Verification items for the finished model (mm, model axes). Give positions to 0.01 mm unless a question says otherwise; leave off trailing zeros. Write each loop counter-clockwise with the first axis right and the second up, starting at its lowest first coordinate (ties: lowest second). Pieces come first, ordered by that corner, then holes.
from build123d import *

# Parameters (mm, degrees)
SKETCH1_W           = 52.3875
SKETCH1_H           = 52.3875
SKETCH1_R           = 9.525
BOSS_EXTRUDE1_DEPTH = 23.8125
FILLET1_R           = 2.54


with BuildPart() as part:
    # Sketch1 → Boss-Extrude1 (new body)
    with BuildSketch(Plane(origin=(0, 0, 0), x_dir=(1, 0, 0), z_dir=(0, 1, 0))):
        Rectangle(SKETCH1_W, SKETCH1_H)
        with Locations(Location((0, 0, 0), (0, 0, 270))):
            Circle(SKETCH1_R, mode=Mode.SUBTRACT)
    extrude(amount=BOSS_EXTRUDE1_DEPTH)

    # Fillet1
    fillet1_edges = [part.edges().sort_by_distance(p)[0] for p in [
        (26.19375, 23.8125, 0),
        (0, 23.8125, -9.525),
        (0, 23.8125, -26.19375),
        (-26.19375, 23.8125, 0),
        (0, 23.8125, 26.19375),
    ]]
    fillet(fillet1_edges, radius=FILLET1_R)


solid = part.part
Item 1: Sectioned sample at C-C on y = 3.5. Record the cut outline in (x, z) (3 decimals).
Answer key:
outline: (-26.194, -26.194) - (26.194, -26.194) - (26.194, 26.194) - (-26.194, 26.194) - close; hole circle Ø19.05 at (0, 0)
Item 2: Sectioned sample at D-D on y = 22. Record the cut outline in (x, z).
Answer key:
outline: (-26.09, -26.09) - (26.09, -26.09) - (26.09, 26.09) - (-26.09, 26.09) - close; hole circle Ø19.26 at (0, 0)
Item 3: Release check for a two-part mould opening along X. For faces 1 (the face through (11, 0, 0)), 2 (the face through (26.194, 10, 0)), 3 (the face through (-5.796, 10.487, -7.559)) record: released by +X, released by -X, zero draft, split by the parting line, or undercut.
Answer key:
face 1: zero draft
face 2: released by +X
face 3: undercut
Item 4: Scan lines: line 1 along X through (y, z) = (5.25, 0) (3 decimals); line 2 along X through (y, z) = (21.5, -16.5); line 3 along X through (y, z) = (23, 6.5). Record each from-to range of solid material in increasing order.
Answer key:
line 1: x = -26.194 to -9.525, 9.525 to 26.194
line 2: x = -26.18 to 26.18
line 3: x = -25.52 to -7.86, 7.86 to 25.52
Item 5: Sectioned sample at B-B on z = 0. Record the cut outline in (x, y) (1 decimal), then the cut area to 3 significant figures.
Answer key:
outline: (-26.2, 0) - (-9.5, 0) - (-9.5, 21.3) arc R2.5 ccw to (-12.1, 23.8) - (-23.7, 23.8) arc R2.5 ccw to (-26.2, 21.3) - close; (9.5, 0) - (26.2, 0) - (26.2, 21.3) arc R2.5 ccw to (23.7, 23.8) - (12.1, 23.8) arc R2.5 ccw to (9.5, 21.3) - close
area: 788 mm2
Item 6: Sectioned sample at A-A on x = 0. Record the cut outline in (y, z) (1 decimal), then the cut area to 3 significant figures.
Answer key:
outline: (0, -26.2) - (21.3, -26.2) arc R2.5 ccw to (23.8, -23.7) - (23.8, -12.1) arc R2.5 ccw to (21.3, -9.5) - (0, -9.5) - close; (0, 9.5) - (21.3, 9.5) arc R2.5 ccw to (23.8, 12.1) - (23.8, 23.7) arc R2.5 ccw to (21.3, 26.2) - (0, 26.2) - close
area: 788 mm2
Item 7: Depth check by flat-ended pin: pin 1 (22 mm diameter, centred on x = 0, z = 0, fed in from +Y). Enter the tip coordinate at first touch or a pass-through.
Answer key:
pin 1: stops at y = 23.58
